Read the model definition and answer for the solid it produces. Units are mm, in the model's axes. A direction names the side the tool comes from. Round coordinates to 2 decimals unless told otherwise and drop trailing zeros. Order: outer loops, then holes, each group sorted by start corner. A loop starts at its lowest first (then second) coordinate and runs counter-clockwise, first axis right, second up.
Autodesk Inventor part; units mm, degrees
ref_plane "YZ Plane" through (0, 0, 0) normal (1, 0, 0) x (0, 1, 0)
ref_plane "XZ Plane" through (0, 0, 0) normal (0, 1, 0) x (-1, 0, 0)
ref_plane "XY Plane" through (0, 0, 0) normal (0, 0, 1) x (1, 0, 0)
sketch "Sketch1" plane through (0, 0, 0) normal (0, 1, 0) x (-1, 0, 0)
  line L0 (0, 0) -> (18, 0)
  line L1 (0, 0) -> (0, -5)
  line L2 (0, -5) -> (3.5719, -45.8274)
  line L3 (18, 0) -> (18, -5)
  line L4 (18, -5) -> (7.5719, -46.8247)
  line L5 (3.5719, -45.8274) -> (7.5719, -46.8247)
  dimension "d0" = 18
  dimension "d1" = 5
  dimension "d3" = 175
  dimension "d6" = 76
  dimension "d7" = 4
extrude "Extrusion1" add sketch "Sketch1" along normal blind 5
shell "Shell1" thickness 3.5 removed faces 2 at (-7.1906, 5, -18.6091) at (-7.1906, 0, -18.6091)
fillet "Fillet1" radius 1.5875 5 edges at (-3.5, 2.5, -4.8472) (-6.3393, 2.5, -37.3009) (-3.5, 2.5, -3.5) (-14.5, 2.5, -3.5) (-14.5, 2.5, -4.5703)
sketch "Sketch2" plane through (0, 0, 0) normal (0, -1, 0) x (1, 0, 0)
  line L0 (0, 0) -> (-12, 0)
  line L1 (-12, 0) -> (-12, 24)
  line L2 (-12, 24) -> (0, 24)
  line L3 (0, 24) -> (0, 0)
  line L4 (0, 24) -> (-12, 24)
  line L5 (-12, 24) -> (-12, 29)
  line L6 (-12, 29) -> (0, 29)
  line L7 (0, 29) -> (0, 24)
  line L8 (-12, 0) -> (-18, 0)
  line L9 (-18, 0) -> (-18, 24)
  line L10 (-18, 24) -> (-12, 24)
  line L11 (-12, 24) -> (-12, 0)
  line L12 (-18, 24) -> (-13.7574, 24) construction
  line L13 (-12, 29) -> (-16.8, 29)
  line L14 (-16.8, 29) -> (-18, 27.8)
  line L15 (-18, 27.8) -> (-18, 24)
  dimension "d14" = 24
  dimension "d15" = 5
  dimension "d16" = 12
  dimension "d18" = 6
  dimension "d57" = 1.2
  dimension "d58" = 135
extrude "Extrusion2" add sketch "Sketch2" against normal blind 5 contours L8 L9 L10 L1 | L2 L5 L6 L7 | L10 L15 L14 L13 L5
fillet "Fillet3" radius 1 1 edges at (0, 2.5, 29)
sketch "Sketch4" plane through (0, 5, 0) normal (0, 1, 0) x (1, 0, 0)
  line L0 (-12, -24) -> (-12, 0)
  line L1 (-12, -12) -> (-18, -12)
  line L2 (-18, 5) -> (-18, -29)
  line L3 (0, -24) -> (-12, -24)
  line L4 (-12, 0) -> (0, 0)
  circle A0 centre (-6, -25.8) radius 0.8
  circle A1 centre (-6, 1.8) radius 0.8
  line L5 (0, -28) -> (0, -24)
  point P0 (-18, 1.9304)
  point P1 (-18, -27.8)
  point P2 (-16.8, -29)
  dimension "d31" = 1.6
  dimension "d32" = 27.6
  dimension "d43" = 6
  dimension "d46" = 13.8
hole "Hole1" at (-6, 5, 25.8) at (-6, 5, -1.8) direction (0, -1, 0) diameter 1.567 depth 10 countersink diameter 2.5 countersink angle 90
sketch "Sketch17" plane through (0, 5, 0) normal (0, 1, 0) x (1, 0, 0)
  line L0 (-15.0964, 25.5) -> (0.714, 25.5)
  line L1 (-12, 0) -> (0, 0)
  line L2 (-5.1146, 3.5) -> (-12.7349, 3.5)
  line L3 (0.714, 25.5) -> (-0.9097, 44.0597)
  line L4 (-15.0964, 25.5) -> (-10.3033, 44.7241)
  line L5 (0, 5) -> (-3.5719, 45.8274)
  line L6 (-7.5719, 46.8247) -> (-18, 5)
  line L7 (-4.6811, 48.4754) -> (-4.2422, 48.3659)
  line L8 (-3.5719, 45.8274) -> (-7.5719, 46.8247)
  arc A0 (-0.9097, 44.0597) -> (-4.6811, 48.4754) centre (-5.8907, 43.6239) ccw
  arc A1 (-4.2422, 48.3659) -> (-10.3033, 44.7241) centre (-5.4518, 43.5145) ccw
  point P0 (-8.9248, 3.5)
  point P1 (-4.4629, 48.4157)
  dimension "d152" = 22
  dimension "d153" = 2.498
  dimension "d154" = 2.142
  dimension "d155" = 2.301
  dimension "d156" = 5
extrude "Extrusion13" [suppressed]
sketch "Sketch18" plane through (-15.4653, 7.5, -25.5) normal (0, 0, 1) x (1, 0, 0)
  line L0 (16.1813, -10) -> (16.1813, 0) construction
  line L1 (4.8628, 0) -> (0, 0) construction
  line L2 (16.1813, -10) -> (0, 0) construction
  line L3 (0, -10) -> (0, 0) construction
  line L4 (16.1813, 0) -> (0, -10) construction
  line L5 (23.0907, 2.5) -> (-6.9093, 2.5)
  line L6 (-6.9093, 2.5) -> (-6.9093, -12.5)
  line L7 (-6.9093, -12.5) -> (23.0907, -12.5)
  line L8 (23.0907, -12.5) -> (23.0907, 2.5)
  line L9 (23.0907, 2.5) -> (-6.9093, -12.5) construction
  line L10 (-6.9093, 2.5) -> (23.0907, -12.5) construction
  point P0 (15.4653, -7.5)
  point P1 (8.0907, -5)
  dimension "d161" = 25
  dimension "d162" = 15
extrude "Extrusion14" [suppressed]
combine "Combine8" [suppressed]
extrude "Extrusion15" [suppressed]
combine "Combine9" [suppressed]
combine "Combine10" [suppressed]
sketch "Sketch20" plane through (-15.4653, 7.5, -21.5) normal (0, 0, 1) x (1, 0, 0)
  line L0 (10.1584, -7.5) -> (13.6718, -7.5)
  line L1 (6.1837, -2.5) -> (2.5765, -2.5)
  line L2 (11.871, -7.5) -> (3.871, -7.5)
  line L3 (3.871, -7.5) -> (3.871, -2.5)
  line L4 (3.871, -2.5) -> (11.871, -2.5)
  line L5 (11.871, -2.5) -> (11.871, -7.5)
  circle A0 centre (19.0907, -8.5) radius 1
  line L6 (23.0907, -12.5) -> (-6.9093, -12.5) construction
  circle A1 centre (-2.9093, -1.5) radius 1
  line L7 (23.0907, -12.5) -> (23.0907, 2.5) construction
  line L8 (23.0907, 2.5) -> (-6.9093, 2.5) construction
  line L9 (11.871, -7.5) -> (3.871, -7.5)
  line L10 (3.871, -7.5) -> (3.871, -10)
  line L11 (3.871, -10) -> (11.871, -10)
  line L12 (11.871, -10) -> (11.871, -7.5)
  line L13 (11.871, -2.5) -> (3.871, -2.5)
  line L14 (3.871, -2.5) -> (3.871, 0)
  line L15 (3.871, 0) -> (11.871, 0)
  line L16 (11.871, 0) -> (11.871, -2.5)
  line L17 (-6.9093, 2.5) -> (-6.9093, -12.5)
  point P0 (15.4653, -7.5)
  point P1 (23.0907, -5)
  point P2 (23.0907, -5)
  dimension "d167" = 9.224
  dimension "d168" = 3.5943
  dimension "d171" = 2
  dimension "d173" = 7.5
  dimension "d175" = 4.22
  dimension "d181" = 2.5
  dimension "d185" = 8
  dimension "d186" = 2.5
  dimension "d202" = 15
  dimension "d203" = 11
  dimension "d204" = 3.561
  dimension "d205" = 2
extrude "Extrusion16" [suppressed]
extrude "Extrusion17" [suppressed]
chamfer "Chamfer2" [suppressed]
chamfer "Chamfer3" [suppressed]
chamfer "Chamfer4" [suppressed]
chamfer "Chamfer5" [suppressed]
sketch "Sketch21" plane through (-15.4653, 7.5, -25.5) normal (0, 0, 1) x (1, 0, 0)
  line L0 (23.0907, 2.5) -> (-6.9093, 2.5)
  line L1 (-6.9093, 2.5) -> (-6.9093, -10.5)
  line L2 (23.0907, 2.5) -> (-6.9093, 2.5)
  line L3 (-6.9093, 2.5) -> (-6.9093, -5)
  line L4 (-6.9093, -5) -> (23.0907, -5)
  line L5 (23.0907, -5) -> (23.0907, 2.5)
  point P0 (15.4653, -7.5)
  dimension "d194" = 7.5
extrude "Extrusion18" [suppressed]
extrude "Extrusion19" [suppressed]
combine "Combine11" [suppressed]
sketch "Sketch22" plane through (-15.4653, 7.5, -25.5) normal (0, 0, 1) x (1, 0, 0)
  circle A0 centre (-2.9093, -1.5) radius 1 construction
  line L0 (-2.9093, -2.5) -> (-2.9093, -1.5) construction
  circle A1 centre (-2.9093, -1.5) radius 1
  point P0 (15.4653, -7.5)
extrude "Extrusion20" [suppressed]
chamfer "Chamfer7" [suppressed]
sketch "Sketch23" plane through (7.6254, 10, -60.5) normal (0, 0, -1) x (-1, 0, 0)
  line L0 (30, -7.5) -> (3.5, -7.5)
  line L1 (30, -7.5) -> (30, -11)
  line L2 (26.5, -7.5) -> (30, -11)
  line L3 (30, -11) -> (26.5, -7.5)
  line L4 (26.5, -7.5) -> (30, -7.5)
  line L5 (0, -4) -> (3.5, -7.5)
  line L6 (3.5, -7.5) -> (0, -7.5)
  line L7 (0, -7.5) -> (0, -4)
  line L8 (0, -4) -> (3.5, -7.5)
  point P0 (7.6254, -10)
extrude "Extrusion21" [suppressed]
extrude "Extrusion22" [suppressed]
combine "Combine12" [suppressed]
combine "Combine13" [suppressed]
fillet "Fillet6" [suppressed]
sketch "Sketch24" plane through (-22.3746, 10, -25.5) normal (0, 1, 0) x (1, 0, 0)
  circle A0 centre (24, 29) radius 1
  line L0 (30, 35) -> (0, 35)
  line L1 (30, 0) -> (30, 35)
  circle A1 centre (24, 11) radius 1
  circle A2 centre (6, 29) radius 1
  circle A3 centre (6, 11) radius 1
  point P0 (22.3746, -25.5)
  dimension "d216" = 2
  dimension "d217" = 4.064
  dimension "d218" = 4.147
  dimension "d221" = 18
  dimension "d224" = 20
extrude "Extrusion23" [suppressed]
extrude "Extrusion24" [suppressed]
chamfer "Chamfer8" [suppressed]
chamfer "Chamfer9" [suppressed]
properties part number "CAM3D_3D tisk"
Q1. For a pull along X with two mould halves and no side action, classify faces 4 (the face through (0, 2, -2)), 5 (the face through (-18, 2, 12)), 6 (the face through (-6, 2, 24)), 7 (the face through (-9, 2, -3.5)) as released by +X, released by -X, zero draft, split by the parting line, or undercut.
Outcome:
face 4: released by +X
face 5: released by -X
face 6: zero draft
face 7: undercut
Q2. Straight lines are drawn through the part: probe 1 along X at (y, z) = (2.8, 25.8); probe 2 along Z at (x, y) = (-7, 4.65); probe 3 along Z at (x, y) = (-6, 2.15). For each, find the intervals that lie inside material, in ascending order.
Outcome:
probe 1: x = -18 to -6.78, -5.22 to 0
probe 2: z = -46.68 to -29.3, -3.5 to 0, 24 to 29
probe 3: z = -46.43 to -28.86, -3.5 to -2.58, -1.02 to 0, 24 to 25.02, 26.58 to 29
Q3. A cutting plane is placed at A-A, the plane z = 25.8. Give the vertices of the cut face in (x, y).
Outcome:
outline: (-18, 0) - (-6.78, 0) - (-6.78, 4.53) - (-7.25, 5) - (-18, 5) - close; (-5.22, 0) - (0, 0) - (0, 5) - (-4.75, 5) - (-5.22, 4.53) - close
Q4. A cutting plane is placed at D-D, the plane z = 16.5. Give the vertices of the cut face in (x, y).
Outcome:
outline: (-18, 0) - (-12, 0) - (-12, 5) - (-18, 5) - close
Q5. Flat-ended cylindrical pins translate along their axes: pin 1 (1 mm diameter, centred on y = 1, z = -17.5, fed in from +X); pin 2 (1.5 mm diameter, centred on y = 3, z = 12, fed in from +X); pin 3 (1.5 mm diameter, centred on x = -3, y = 2.5, fed in from -Z). Find the tip coordinate at first contact, or state that the pin passes through.
Outcome:
pin 1: stops at x = -1.05
pin 2: stops at x = -12
pin 3: stops at z = -45.87
Q6. A cutting plane is placed at B-B, the plane z = -24. Give the vertices of the cut face in (x, y).
Outcome:
outline: (-13.26, 0) - (-9.66, 0) - (-9.66, 5) - (-13.26, 5) - close; (-5.18, 0) - (-1.66, 0) - (-1.66, 5) - (-5.18, 5) - close
Q7. For faces 1 (the face through (-11.5, 2.5, -16.6)), 2 (the face through (-9, 2, 29)), 3 (the face through (-6, 2, 0)), determine the directions among +Z, -Z, +X, -X, +Y, -Y from which every point of the face is accessible in a straight line to the end or side of a thin tool.
Outcome:
face 1: +Y, -Y
face 2: +Z, +X, -X, +Y, -Y
face 3: +X, +Y, -Y
Q8. A cutting plane is placed at C-C, the plane y = 3.5. Give the number of separate pieces and of enclosed holes in the cut face, plus the area to 3 significant figures.
Outcome:
separate pieces: 1
enclosed holes: 3
area: 596 mm2
